from build123d import *

# Parameters (mm, degrees)
BOSS_EXTRUDE1_DEPTH = 13
SKETCH2_R           = 3.984832534
CUT_EXTRUDE1_DEPTH  = 70.384008424


with BuildPart() as part:
    # Sketch1 → Boss-Extrude1 (new body)
    with BuildSketch(Plane(origin=(0, 0, 0), x_dir=(1, 0, 0), z_dir=(0, 1, 0))):
        with BuildLine():
            Line((-26.375, -61.5), (26.375, -61.5))
            ThreePointArc((26.375, -61.5), (28.496320344, -60.621320344), (29.375, -58.5))
            Line((29.375, -58.5), (29.375, 61.5))
            Line((29.375, 61.5), (-29.375, 61.5))
            Line((-29.375, 61.5), (-29.375, -58.5))
            ThreePointArc((-29.375, -58.5), (-28.496320344, -60.621320344), (-26.375, -61.5))
        make_face()
    extrude(amount=BOSS_EXTRUDE1_DEPTH)

    # Sketch2 → Cut-Extrude1 (cut, through all)
    with BuildSketch(Plane(origin=(0, 13, 0), x_dir=(1, 0, 0), z_dir=(0, 1, 0))):
        with Locations(Location((-21.724826846, 52.625202096, 0), (0, 0, 270))):
            Circle(SKETCH2_R)
    extrude(amount=-CUT_EXTRUDE1_DEPTH, mode=Mode.SUBTRACT)


solid = part.part
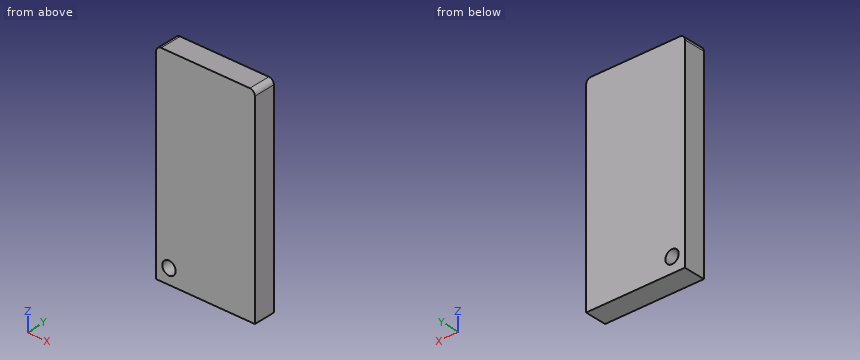
Check sheet for the modelled part. Datum: model origin and axes. Units: mm. Give positions to 0.01 mm unless a question says otherwise; leave off trailing zeros. Order: outer loops, then holes, each group sorted by start corner. A loop starts at its lowest first (then second) coordinate and runs counter-clockwise, first axis right, second up. Notation, with made-up numbers: (-24, 24) - (12, 24) arc R18 ccw to (12, 41) - close; hole circle Ø2 at (7.5, 42). An arc over 180 degrees is marked (long way). Answer as CSV lines item,"result".
1. Section check B-B (z = -50). Record the boundary of the cut face in (x, y) (3 decimals), then the cut area to 3 significant figures.
Result sheet:
outline,"(-29.375, 0) - (-24.723, 0) - (-24.723, 13) - (-29.375, 13) - close; (-18.727, 0) - (29.375, 0) - (29.375, 13) - (-18.727, 13) - close"
area,"686 mm²"
2. Section check A-A (x = -20). Record the boundary of the cut face in (y, z).
Result sheet:
outline,"(0, -61.5) - (13, -61.5) - (13, -56.22) - (0, -56.22) - close; (0, -49.03) - (13, -49.03) - (13, 61.5) - (0, 61.5) - close"
3. Scan lines: probe 1 along Z at (x, y) = (-21.5, 5); probe 2 along X at (y, z) = (2, -50) (3 decimals); probe 3 along Z at (x, y) = (-20.5, 12). Record each from-to range of solid material in increasing order. Write a range as from..to.
Result sheet:
probe 1,"-61.5..-56.6, -48.65..61.5"
probe 2,"-29.375..-24.723, -18.727..29.375"
probe 3,"-61.5..-56.42, -48.83..61.5"
